```python
from build123d import *

# Parameters (mm, degrees)
CROQUIS1_R              = 3.7
SALIENTE_EXTRUIR2_DEPTH = 4.3
CROQUIS2_R              = 2.5
CORTAR_EXTRUIR1_DEPTH   = 1.5
CORTAR_EXTRUIR2_START   = -1
CROQUIS3_R              = 2.5
CORTAR_EXTRUIR2_DEPTH   = 1
CROQUIS4_R              = 1
CORTAR_EXTRUIR3_DEPTH   = 1.8
SALIENTE_EXTRUIR3_DEPTH = 1.8
CROQUIS6_R              = 0.595
CORTAR_EXTRUIR4_DEPTH   = 1.8
SKETCH1_R               = 2.5
BOSS_EXTRUDE1_DEPTH     = 10
SKETCH2_W               = 25.5
SKETCH2_H               = 2.3
CUT_EXTRUDE1_DEPTH      = 7


with BuildPart() as part:
    # Croquis1 → Saliente-Extruir2 (new body)
    with BuildSketch(Plane(origin=(0, 0, 0), x_dir=(1, 0, 0), z_dir=(0, 1, 0))):
        with Locations(Location((0, 0, 0), (0, 0, 90))):
            Circle(CROQUIS1_R)
    extrude(amount=SALIENTE_EXTRUIR2_DEPTH)

    # Croquis2 → Cortar-Extruir1 (cut)
    with BuildSketch(Plane.XZ):
        with Locations(Location((0, 0, 0), (0, 0, 270))):
            Circle(CROQUIS2_R)
    extrude(amount=-CORTAR_EXTRUIR1_DEPTH, mode=Mode.SUBTRACT)

    # Croquis3 → Cortar-Extruir2 (cut)
    with BuildSketch(Plane(origin=(0, 4.3, 0), x_dir=(1, 0, 0), z_dir=(0, 1, 0)).offset(CORTAR_EXTRUIR2_START)):
        with Locations(Location((0, 0, 0), (0, 0, 90))):
            Circle(CROQUIS3_R)
    extrude(amount=CORTAR_EXTRUIR2_DEPTH, mode=Mode.SUBTRACT)

    # Croquis4 → Cortar-Extruir3 (cut)
    with BuildSketch(Plane(origin=(0, 3.3, 0), x_dir=(1, 0, 0), z_dir=(0, 1, 0))):
        with Locations(Location((0, 0, 0), (0, 0, 270))):
            Circle(CROQUIS4_R)
    extrude(amount=-CORTAR_EXTRUIR3_DEPTH, mode=Mode.SUBTRACT)

    # Croquis5 → Saliente-Extruir3 (add)
    with BuildSketch(Plane(origin=(0, 4.3, 0), x_dir=(1, 0, 0), z_dir=(0, 1, 0))):
        with BuildLine():
            Line((-2.16564, 3.000000565), (-3.120237459, 0))
            Line((-3.120237459, 0), (-2.16564, -3.000000565))
            Line((-2.16564, -3.000000565), (-14.3, -2))
            ThreePointArc((-14.3, -2), (-16.3, 0), (-14.3, 2))
            Line((-14.3, 2), (-2.16564, 3.000000565))
        make_face()
        with BuildLine():
            Line((3.120237459, 0), (2.16564, -3.000000565))
            Line((2.16564, -3.000000565), (14.3, -2))
            ThreePointArc((14.3, -2), (16.3, 0), (14.3, 2))
            Line((14.3, 2), (2.16564, 3.000000565))
            Line((2.16564, 3.000000565), (3.120237459, 0))
        make_face()
    extrude(amount=-SALIENTE_EXTRUIR3_DEPTH)

    # Croquis6 → Cortar-Extruir4 (cut)
    with BuildSketch(Plane(origin=(0, 4.3, 0), x_dir=(1, 0, 0), z_dir=(0, 1, 0))):
        with Locations(Location((-14.705, 0, 0), (0, 0, 270))):
            Circle(CROQUIS6_R)
        with Locations(Location((-12.705, 0, 0), (0, 0, 270))):
            Circle(CROQUIS6_R)
        with Locations(Location((-10.705, 0, 0), (0, 0, 270))):
            Circle(CROQUIS6_R)
        with Locations(Location((-8.705, 0, 0), (0, 0, 270))):
            Circle(CROQUIS6_R)
        with Locations(Location((-6.705, 0, 0), (0, 0, 270))):
            Circle(CROQUIS6_R)
        with Locations(Location((-4.705, 0, 0), (0, 0, 270))):
            Circle(CROQUIS6_R)
        with Locations(Location((14.705, 0, 0), (0, 0, 90))):
            Circle(CROQUIS6_R)
        with Locations(Location((12.705, 0, 0), (0, 0, 90))):
            Circle(CROQUIS6_R)
        with Locations(Location((10.705, 0, 0), (0, 0, 90))):
            Circle(CROQUIS6_R)
        with Locations(Location((8.705, 0, 0), (0, 0, 90))):
            Circle(CROQUIS6_R)
        with Locations(Location((6.705, 0, 0), (0, 0, 90))):
            Circle(CROQUIS6_R)
        with Locations(Location((4.705, 0, 0), (0, 0, 90))):
            Circle(CROQUIS6_R)
    extrude(amount=-CORTAR_EXTRUIR4_DEPTH, mode=Mode.SUBTRACT)

    # Sketch1 → Boss-Extrude1 (add)
    with BuildSketch(Plane(origin=(0, 4.3, 0), x_dir=(1, 0, 0), z_dir=(0, 1, 0))):
        with BuildLine():
            Line((2.16564, -3.000000565), (14.3, -2))
            ThreePointArc((14.3, -2), (16.3, 0), (14.3, 2))
            Line((14.3, 2), (2.16564, 3.000000565))
            ThreePointArc((2.16564, 3.000000565), (0, 3.7), (-2.16564, 3.000000565))
            Line((-2.16564, 3.000000565), (-14.3, 2))
            ThreePointArc((-14.3, 2), (-16.3, 0), (-14.3, -2))
            Line((-14.3, -2), (-2.16564, -3.000000565))
            ThreePointArc((-2.16564, -3.000000565), (0, -3.7), (2.16564, -3.000000565))
        make_face()
        with Locations(Location((0, 0, 0), (0, 0, 90))):
            Circle(SKETCH1_R, mode=Mode.SUBTRACT)
    extrude(amount=BOSS_EXTRUDE1_DEPTH)

    # Sketch2 → Cut-Extrude1 (cut)
    with BuildSketch(Plane(origin=(0, 14.3, 0), x_dir=(1, 0, 0), z_dir=(0, 1, 0))):
        Rectangle(SKETCH2_W, SKETCH2_H)
    extrude(amount=-CUT_EXTRUDE1_DEPTH, mode=Mode.SUBTRACT)


solid = part.part
```
Geometry check sheet. Reference: the model listing, model coordinates, mm. A direction names the side the tool comes from. Round coordinates to 2 decimals unless told otherwise and drop trailing zeros. Write each loop counter-clockwise with the first axis right and the second up, starting at its lowest first coordinate (ties: lowest second). Pieces come first, ordered by that corner, then holes. Notation, with made-up numbers: (13, 81) -> (71, 81) arc R11 cw to (71, 100) -> close; hole circle Ø1 at (16.25, -22). An arc over 180 degrees is marked (long way). Put each result on its own line as item: value.
1) Cross-section at B-B, the plane x = -1.5. Enter the section's corners in (y, z), plus the area to 3 significant figures.
Recorded:
outline: (0, -3.38) -> (14.3, -3.38) -> (14.3, -2) -> (3.3, -2) -> (3.3, 2) -> (14.3, 2) -> (14.3, 3.38) -> (0, 3.38) -> (0, 2) -> (1.5, 2) -> (1.5, -2) -> (0, -2) -> close
area: 46.7 mm2
2) Thickness scan on probe 1 along X at (y, z) = (8.5, 0); probe 2 along Z at (x, y) = (-3, 11.5); probe 3 along Z at (x, y) = (-12, 10). Record the ranges inside material, lowest first. Write a range as from..to.
Recorded:
probe 1: x = -16.3..-12.75, 12.75..16.3
probe 2: z = -2.93..-1.15, 1.15..2.93
probe 3: z = -2.19..-1.15, 1.15..2.19
3) Depth check by flat-ended pin: P1, Ø1.3, axis at x = -9, z = 0, coming from the -Y side; P2, Ø0.7, axis at x = -7, z = 0, coming from the +Y side; P3, Ø0.6, axis at x = 8.5, z = 0, coming from the -Y side. Enter the tip coordinate at first touch or a pass-through.
Recorded:
P1: stops at y = 2.5
P2: stops at y = 7.3
P3: stops at y = 4.3
4) Release check for a two-part mould opening along X. For faces 4 (the face through (12.75, 11, 0)), 5 (the face through (0, 14.3, -3)), 6 (the face through (8.318, 8.317, -2.493)) record: pulls with the +X half, pulls with the -X half, needs draft (parallel to the pull), parting line crosses it, or undercut.
Recorded:
face 4: undercut
face 5: needs draft
face 6: pulls with the +X half
5) Access from +Z, -Z, +X, -X, +Y, -Y to the whole of each face (thin tool, end or side, straight path). Record for faces 1 (the face through (-3, 0, 0)), 2 (the face through (-2.44, 0.74, 0.54)), 3 (the face through (-8, 7.3, 0)).
Recorded:
face 1: +Z, -Z, +X, -X, -Y
face 2: -Y
face 3: +Y
6) Cross-section at D-D, the plane x = -5. Enter the section's corners in (y, z), plus the area to 3 significant figures.
Recorded:
outline: (2.5, -2.77) -> (14.3, -2.77) -> (14.3, -1.15) -> (7.3, -1.15) -> (7.3, 1.15) -> (14.3, 1.15) -> (14.3, 2.77) -> (2.5, 2.77) -> (2.5, 0.52) -> (4.3, 0.52) -> (4.3, -0.52) -> (2.5, -0.52) -> close
area: 47.3 mm2
7) Cross-section at A-A, the plane y = 10. Enter the section's corners in (x, z).
Recorded:
outline: (-14.3, -2) -> (-2.17, -3) arc R3.7 ccw to (2.17, -3) -> (14.3, -2) arc R2 ccw to (14.3, 2) -> (2.17, 3) arc R3.7 ccw to (-2.17, 3) -> (-14.3, 2) arc R2 ccw to start; hole (-12.75, -1.15) -> (-2.22, -1.15) arc R2.5 ccw to (2.22, -1.15) -> (12.75, -1.15) -> (12.75, 1.15) -> (2.22, 1.15) arc R2.5 ccw to (-2.22, 1.15) -> (-12.75, 1.15) -> close
8) Cross-section at C-C, the plane z = 1.5. Enter the section's corners in (x, y).
Recorded:
outline: (-15.62, 2.5) -> (-3.38, 2.5) -> (-3.38, 0) -> (-2, 0) -> (-2, 1.5) -> (2, 1.5) -> (2, 0) -> (3.38, 0) -> (3.38, 2.5) -> (15.62, 2.5) -> (15.62, 14.3) -> (2, 14.3) -> (2, 3.3) -> (-2, 3.3) -> (-2, 14.3) -> (-15.62, 14.3) -> close
